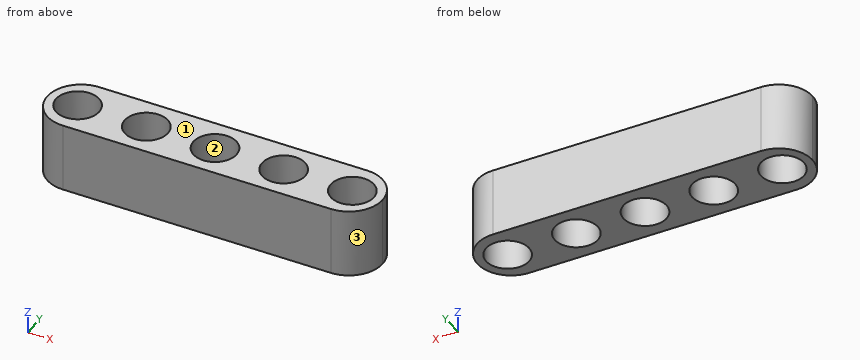
Autodesk Inventor part; units mm, degrees
ref_plane "YZ Plane" through (0, 0, 0) normal (1, 0, 0) x (0, 1, 0)
ref_plane "XZ Plane" through (0, 0, 0) normal (0, 1, 0) x (-1, 0, 0)
ref_plane "XY Plane" through (0, 0, 0) normal (0, 0, 1) x (1, 0, 0)
sketch "Sketch1" plane through (0, 0, 0) normal (0, 0, 1) x (1, 0, 0)
  line L0 (0, 0) -> (39, 0)
  line L1 (39, 0) -> (39, -7.8)
  line L2 (39, -7.8) -> (0, -7.8)
  line L3 (0, -7.8) -> (0, 0)
  dimension "d0" = 39
  dimension "d1" = 7.8
extrude "Extrusion1" add sketch "Sketch1" along normal blind 8
fillet "Fillet1" radius 3.9 1 edges at (0, 0, 4)
fillet "Fillet2" radius 3.9 1 edges at (0, -7.8, 4)
fillet "Fillet3" radius 3.9 1 edges at (39, -7.8, 4)
fillet "Fillet4" radius 3.9 1 edges at (39, 0, 4)
sketch "Sketch2" plane through (0, 0, 8) normal (0, 0, 1) x (1, 0, 0)
  line L0 (35.1, 0) -> (3.9, 0)
  arc A0 (35.1, -7.8) -> (35.1, 0) centre (35.1, -3.9) ccw
  line L1 (0, -3.9) -> (39, -3.9)
  circle A1 centre (19.5, -3.9) radius 2.5
  circle A2 centre (27.5, -3.9) radius 2.5
  circle A3 centre (35.5, -3.9) radius 2.5
  circle A4 centre (11.5, -3.9) radius 2.5
  circle A5 centre (3.5, -3.9) radius 2.5
  point P0 (0, 0)
  dimension "d16" = 39
  dimension "d17" = 5
  dimension "d18" = 5
  dimension "d19" = 5
  dimension "d20" = 5
  dimension "d21" = 5
  dimension "d24" = 3
  dimension "d25" = 3
  dimension "d27" = 3
  dimension "d28" = 3
extrude "Extrusion2" cut sketch "Sketch2" against normal blind 8
properties part number "Transmission_Holder_5_Place_Holder"
The model under review builds one solid part; all positions refer to its coordinate system, in mm. Face numbers are marked on the shaded views. Give positions to 0.01 mm unless a question says otherwise; leave off trailing zeros. Loops run counter-clockwise (first coordinate to the right, second up) from the corner with the lowest first, then second, coordinate; pieces in that order, holes last. Notation, with made-up numbers: (52.25, 10.25) - (104.25, 10.25) arc R20 ccw to (104.25, 36.25) - close; hole circle Ø6 at (-8, 21). An arc over 180 degrees is marked (long way). Answer as a JSON object with one key per item and string values.
Q1. Insertion check: pin 1 (2 mm diameter, centred on y = -1, z = 7, fed in from -X). The pin has a flat end and moves straight along its axis. Give the tip position at first contact, or say it passes through.
Worked out:
{"pin 1": "stops at x = 0.49"}
Q2. Add section C-C on y = -2. State the section outline as (x, z) points.
Worked out:
{"outline": "(0.49, 0) - (1.88, 0) - (1.88, 8) - (0.49, 8) - close; (5.12, 0) - (9.88, 0) - (9.88, 8) - (5.12, 8) - close; (13.12, 0) - (17.88, 0) - (17.88, 8) - (13.12, 8) - close; (21.12, 0) - (25.88, 0) - (25.88, 8) - (21.12, 8) - close; (29.12, 0) - (33.88, 0) - (33.88, 8) - (29.12, 8) - close; (37.12, 0) - (38.51, 0) - (38.51, 8) - (37.12, 8) - close"}
Q3. Add section B-B on x = 11.5. State the section outline as (y, z) points.
Worked out:
{"outline": "(-7.8, 0) - (-6.4, 0) - (-6.4, 8) - (-7.8, 8) - close; (-1.4, 0) - (0, 0) - (0, 8) - (-1.4, 8) - close"}
Q4. Add section D-D on x = 19. State the section outline as (y, z) points, plus the area to 3 significant figures.
Worked out:
{"outline": "(-7.8, 0) - (-6.35, 0) - (-6.35, 8) - (-7.8, 8) - close; (-1.45, 0) - (0, 0) - (0, 8) - (-1.45, 8) - close", "area": "23.2 mm^2"}
Q5. To check wall thickness, follow line 1 along X through (y, z) = (-3.9, 4); line 2 along Y through (x, z) = (11.5, 5.5); line 3 along X through (y, z) = (-5.25, 6.5). State the ranges of each line that lie inside material, in increasing order.
Worked out:
{"line 1": "x = 0 to 1, 6 to 9, 14 to 17, 22 to 25, 30 to 33, 38 to 39", "line 2": "y = -7.8 to -6.4, -1.4 to 0", "line 3": "x = 0.24 to 1.4, 5.6 to 9.4, 13.6 to 17.4, 21.6 to 25.4, 29.6 to 33.4, 37.6 to 38.76"}
Q6. Mouldability with a two-part tool opening along X and no side actions: class the marked faces 1, 2 and 3 as +X half, -X half, draft (parallel to the pull), parting line (faces both ways), or undercut.
Worked out:
{"face 1": "draft", "face 2": "undercut", "face 3": "+X half"}
Q7. Add section A-A on z = 1.25. Count the separate pieces of the cut face and the enclosed holes in it, plus the area to 3 significant figures.
Worked out:
{"separate pieces": "1", "enclosed holes": "5", "area": "193 mm^2"}
